Here's how the part is built. I have some questions about the finished solid (model axes, mm). Face numbers are marked on the shaded views. A direction names the side the tool comes from. Round coordinates to 2 decimals unless told otherwise and drop trailing zeros. Loops run counter-clockwise (first coordinate to the right, second up) from the corner with the lowest first, then second, coordinate; pieces in that order, holes last. Notation, with made-up numbers: (55, 77.25) -> (76, 77.25) arc R25 ccw to (76, 103.25) -> close; hole circle Ø4 at (-10, -14.5). An arc over 180 degrees is marked (long way). Use one line per item in the form item = value. Start each with the question number.
Item 1: If we section it at D-D (z = 8.25): Write out the boundary of the cut face in (x, y), then the cut area to 3 significant figures.
Item 2: If I drill on L1, parallel to Y at x = 0, z = 4.45; L2, parallel to X at y = 0.5, z = 9.5, over which ranges is the centre line in solid material (lowest first)? Write a range as [from, to].
Item 3: If we section it at A-A (x = 0): Write out the boundary of the cut face in (y, z), then the cut area to 3 significant figures.
Item 4: If we section it at B-B (y = 0): Write out the boundary of the cut face in (x, z).
Item 5: I'm going to push flat-ended pins straight in: pin 1 Ø0.5 at (x, z) = (2, 0.5) entering from +Y; pin 2 Ø3 at (x, y) = (0, 0) entering from -Z; pin 3 Ø1.5 at (x, z) = (0, 23) entering from -Y. Where does each tip first touch, or does it pass through?
Item 6: For the marked faces 1 and 2, which set-ups out of +Z, -Z, +X, -X, +Y, -Y let a thin tool reach every point of the face, with its end or its side?
Item 7: If we section it at C-C (z = 22.25): Write out the boundary of the cut face in (x, y).
Autodesk Inventor part; units mm, degrees
ref_plane "YZ Plane" through (0, 0, 0) normal (1, 0, 0) x (0, 1, 0)
ref_plane "XZ Plane" through (0, 0, 0) normal (0, 1, 0) x (-1, 0, 0)
ref_plane "XY Plane" through (0, 0, 0) normal (0, 0, 1) x (1, 0, 0)
sketch "Sketch1" plane through (0, 0, 0) normal (0, 1, 0) x (-1, 0, 0)
  line L0 (0, 0) -> (-3, 0)
  line L1 (-3, 0) -> (-3, 20)
  line L2 (-3, 20) -> (-1.5, 20)
  line L3 (-1.5, 20) -> (-1.5, 26)
  line L4 (-1.5, 26) -> (0, 26)
  line L5 (0, 26) -> (0, 0)
  dimension "d1" = 6
  dimension "d2" = 20
  dimension "d3" = 3
  dimension "d4" = 6
revolve "Revolution1" add sketch "Sketch1" angle 360 about axis through (0, 0, 26) along (0, 0, -1)
sketch "Sketch2" plane through (0, 0, 0) normal (0, 0, -1) x (-1, 0, 0)
  line L0 (-3, -0.5) -> (3, -0.5)
  line L1 (3, -0.5) -> (3, 0.5)
  line L2 (3, 0.5) -> (-3, 0.5)
  line L3 (-3, 0.5) -> (-3, -0.5)
  line L4 (-3, -0.5) -> (3, 0.5) construction
  line L5 (3, -0.5) -> (-3, 0.5) construction
  circle A0 centre (0, 0) radius 3
  dimension "d6" = 1
extrude "Extrusion1" cut sketch "Sketch2" against normal blind 1 contours L3 A0 L0 | A0 L2 L0 | L3 L2 A0 | A0 L1 L0 | A0 L2 L1
hole "Hole1" at (0, 0, 0) direction (0, 0, 1) diameter 2.459 depth 6
thread "Thread1"
chamfer "Chamfer1" distance 0.3 angle 45 7 edges at (-3, 0, 20) (0, 3, 0) (0, -3, 0) (0, -1.2295, 0) (-0.6697, 1.0311, 0) (0.6697, 1.0311, 0) (-1.5, 0, 26)
properties part number "BRU-320S" material "Stainless Steel AISI 304"
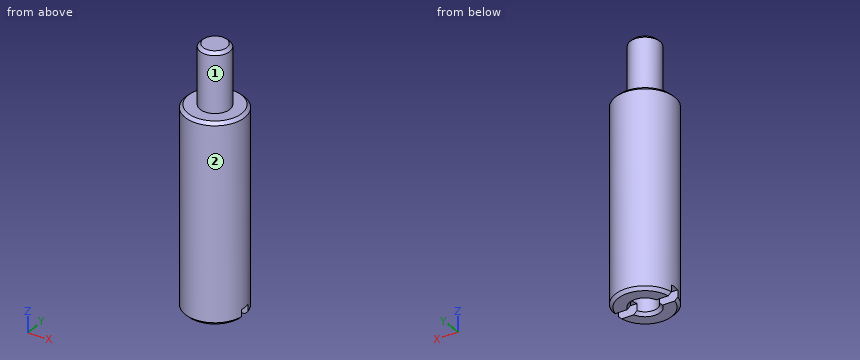
Values found:
q1.outline = circle Ø6 at (0, 0)
q1.area = 28.3 mm2
q2.L1 = [-3, -1.23], [1.23, 3]
q2.L2 = [-2.96, 2.96]
q3.outline = (-3, 0.3) -> (-2.7, 0) -> (-1.53, 0) -> (-1.23, 0.3) -> (-1.23, 6) -> (1.23, 6) -> (1.23, 0.3) -> (1.53, 0) -> (2.7, 0) -> (3, 0.3) -> (3, 19.7) -> (2.7, 20) -> (1.5, 20) -> (1.5, 25.7) -> (1.2, 26) -> (-1.2, 26) -> (-1.5, 25.7) -> (-1.5, 20) -> (-2.7, 20) -> (-3, 19.7) -> close
q3.area = 123 mm2
q4.outline = (-3, 1) -> (-1.23, 1) -> (-1.23, 6) -> (1.23, 6) -> (1.23, 1) -> (3, 1) -> (3, 19.7) -> (2.7, 20) -> (1.5, 20) -> (1.5, 25.7) -> (1.2, 26) -> (-1.2, 26) -> (-1.5, 25.7) -> (-1.5, 20) -> (-2.7, 20) -> (-3, 19.7) -> close
q5.pin_1 = 2.44
q5.pin_2 = 0.03
q5.pin_3 = -1.5
q6.face_1 = +Z
q6.face_2 = +Z, -Z
q7.outline = circle Ø3 at (0, 0)
